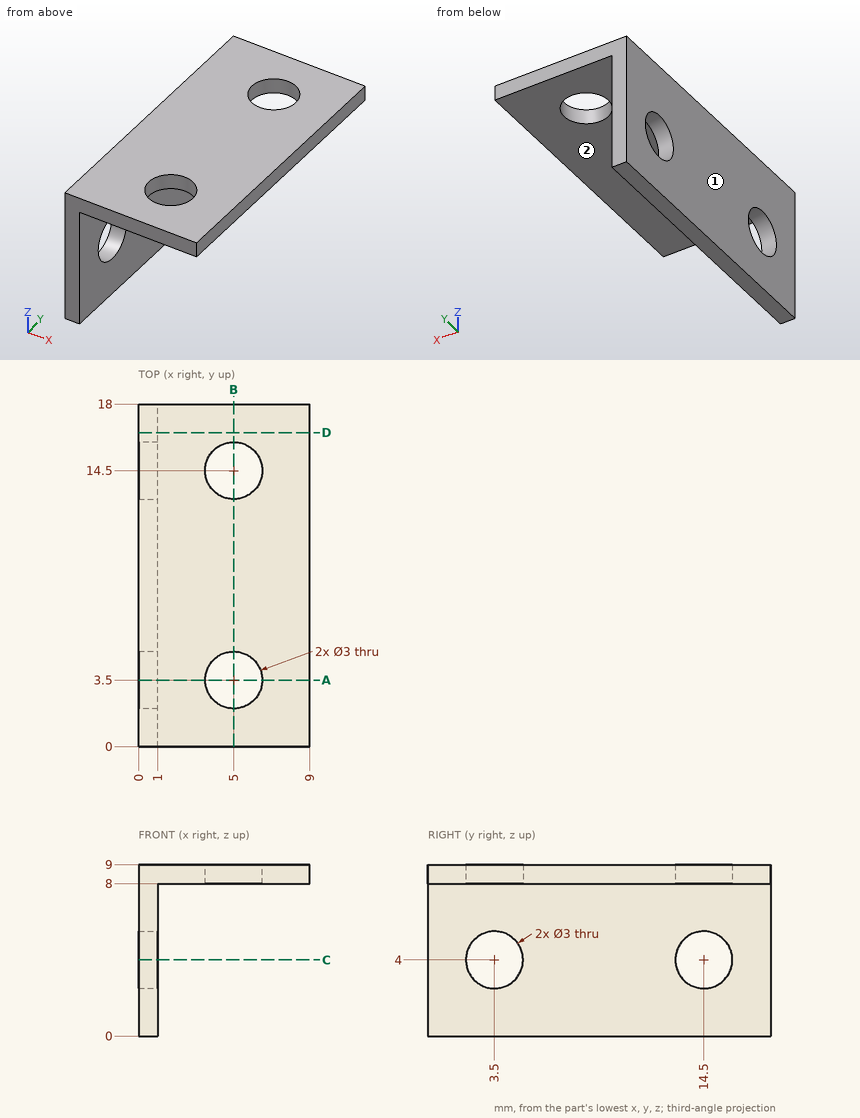
Can you work these out from the drawing? Everything is in mm from the part's minimum corner. A direction names the side the tool comes from. Coordinates: 2 decimals unless noted, no trailing zeros. Loops run counter-clockwise (first coordinate to the right, second up) from the corner with the lowest first, then second, coordinate; pieces in that order, holes last.
1) Imagine slicing it at A-A (y = 3.5). List the corners of the cut face in (x, z) for me, and give its area (3 significant figures).
Reported:
outline: (0, 0) - (1, 0) - (1, 2.5) - (0, 2.5) - close; (0, 5.5) - (1, 5.5) - (1, 8) - (3.5, 8) - (3.5, 9) - (0, 9) - close; (6.5, 8) - (9, 8) - (9, 9) - (6.5, 9) - close
area: 11.0 mm2
2) Please list where these lines run through material, in increasing order: line 1 along Y through (x, z) = (5, 8.6); line 2 along X through (y, z) = (14.5, 8.55); line 3 along Y through (x, z) = (4, 8.75).
Reported:
line 1: y = 0 to 2, 5 to 13, 16 to 18
line 2: x = 0 to 3.5, 6.5 to 9
line 3: y = 0 to 2.38, 4.62 to 13.38, 15.62 to 18
3) Which directions (+Z, -Z, +X, -X, +Y, -Y) give clear straight access to the entire face, cutting with the end or side of a thin tool? Please do the marked faces 1 and 2.
Reported:
face 1: +Z, -Z, -X, +Y, -Y
face 2: -Z, +X, +Y, -Y
4) Imagine slicing it at C-C (z = 4). List the corners of the cut face in (x, y) for me.
Reported:
outline: (0, 0) - (1, 0) - (1, 2) - (0, 2) - close; (0, 5) - (1, 5) - (1, 13) - (0, 13) - close; (0, 16) - (1, 16) - (1, 18) - (0, 18) - close
5) Imagine slicing it at D-D (y = 16.5). List the corners of the cut face in (x, z) for me.
Reported:
outline: (0, 0) - (1, 0) - (1, 8) - (9, 8) - (9, 9) - (0, 9) - close
6) Imagine slicing it at B-B (x = 5). List the corners of the cut face in (y, z) for me, and give its area (3 significant figures).
Reported:
outline: (0, 8) - (2, 8) - (2, 9) - (0, 9) - close; (5, 8) - (13, 8) - (13, 9) - (5, 9) - close; (16, 8) - (18, 8) - (18, 9) - (16, 9) - close
area: 12.0 mm2
7) Will these pins go through, and if not, where does the flat tip stop? pin 1 Ø4 at (y, z) = (13.5, 5) entering from +X; pin 2 Ø2.5 at (x, y) = (6, 7.5) entering from -Z; pin 3 Ø1.8 at (x, y) = (5, 14.5) entering from -Z.
Reported:
pin 1: stops at x = 1
pin 2: stops at z = 8
pin 3: passes through
